Model file for the job. Use its own axes, mm. A direction names the side the tool comes from. Give positions to 0.01 mm unless a question says otherwise; leave off trailing zeros. Order: outer loops, then holes, each group sorted by start corner. A loop starts at its lowest first (then second) coordinate and runs counter-clockwise, first axis right, second up. Notation, with made-up numbers: (1, 7) -> (56, 7) arc R24 ccw to (56, 17) -> close; hole circle Ø7 at (-38.75, 62.5). An arc over 180 degrees is marked (long way). Use CSV: the item, a comma, the result in double quotes. Start each with the question number.
1. Cut at B-B on z = 2.75. List the corners of the cut face in (x, y), then the cut area to 3 significant figures.
2. Drop flat-ended pins along their axis: pin 1 (8 mm diameter, centred on x = 1, y = 5, fed in from -Z); pin 2 (7 mm diameter, centred on y = 12.5, z = 9, fed in from +X); pin 3 (6 mm diameter, centred on x = 5.5, z = 6, fed in from -Y). Give the stop position or say it passes through.
3. Cut at A-A on y = 1.75. List the corners of the cut face in (x, z), then the cut area to 3 significant figures.
4. Wall check: line 1 (X direction, y = 14.75, z = 7.5); line 2 (Z direction, x = 11.25, y = 17.75); line 3 (Y direction, x = 3, z = 2). Give the ranges that are in metal, low to high. Write a range as from..to.
5. 3-axis set-ups, long thin cutter, end or side, ignore diameter. For faces 1 (the flat face through (1, 11, -3)), 2 (the flat face through (6, 0, 7)), 3 (the flat face through (12, 9, 7)), 4 (the flat face through (6, 19, 7)), 5 (the flat face through (-1, 10, -2)): which of +Z, -Z, +X, -X, +Y, -Y reach the whole face in a straight line?
```python
from build123d import *

# Parameters (mm, degrees)
SKETCH1_W           = 12
SKETCH1_H           = 19
BOSS_EXTRUDE1_DEPTH = 14
SKETCH2_W           = 15
SKETCH2_H           = 21
BOSS_EXTRUDE2_DEPTH = 2
BOSS_EXTRUDE3_START = 1
BOSS_EXTRUDE3_DEPTH = 10


with BuildPart() as part:
    # Sketch1 → Boss-Extrude1 (new body)
    with BuildSketch(Plane.XY):
        with Locations((6, 9.5)):
            Rectangle(SKETCH1_W, SKETCH1_H)
    extrude(amount=BOSS_EXTRUDE1_DEPTH)

    # Sketch2 → Boss-Extrude2 (add)
    with BuildSketch(Plane.XY):
        with Locations((6, 9.5)):
            Rectangle(SKETCH2_W, SKETCH2_H)
    extrude(amount=-BOSS_EXTRUDE2_DEPTH)

    # Sketch3 → Boss-Extrude3 (add)
    with BuildSketch(Plane(origin=(0, 0, 0), x_dir=(0, 0, -1), z_dir=(1, 0, 0)).offset(BOSS_EXTRUDE3_START)):
        with BuildLine():
            Line((2, 16.5), (2, 2.5))
            add(Edge.make_bspline(
                [(2, 2.5), (2, 3.412146721), (5.218686286, 14.113667424), (5.401393948, 12.681295538), (2, 16.5)],
                knots=[0, 0, 0, 0, 0.602336799, 1, 1, 1, 1], degree=3))
        make_face()
    extrude(amount=BOSS_EXTRUDE3_DEPTH)


solid = part.part
```
Verdict:
1,outline,"(0, 0) -> (12, 0) -> (12, 19) -> (0, 19) -> close"
1,area,"228 mm^2"
2,pin 1,"z = -3.76"
2,pin 2,"x = 12"
2,pin 3,"y = 0"
3,outline,"(-1.5, -2) -> (13.5, -2) -> (13.5, 0) -> (12, 0) -> (12, 14) -> (0, 14) -> (0, 0) -> (-1.5, 0) -> close"
3,area,"198 mm^2"
4,line 1,"0..12"
4,line 2,"-2..14"
4,line 3,"0..19"
5,face 1,"-Z, -X, +Y, -Y"
5,face 2,"+Z, +X, -X, -Y"
5,face 3,"+Z, +X, +Y, -Y"
5,face 4,"+Z, +X, -X, +Y"
5,face 5,"-Z"
